Geometry check sheet. Reference: the model listing, model coordinates, mm. Round coordinates to 2 decimals unless told otherwise and drop trailing zeros. Loops run counter-clockwise (first coordinate to the right, second up) from the corner with the lowest first, then second, coordinate; pieces in that order, holes last. Notation, with made-up numbers: (-26.75, -9) - (24.25, -9) arc R9 ccw to (24.25, 3) - close; hole circle Ø7 at (-12, -6). An arc over 180 degrees is marked (long way). Answer as CSV lines item,"result". Start each with the question number.
1) Cross-section at A-A on y = 717.5. Record the boundary of the cut face in (x, z), and give its area (3 significant figures).
2) Depth check by flat-ended pin: P1, Ø5, axis at x = 27, z = 10.5, coming from the -Y side; P2, Ø5, axis at y = 1666.5, z = 7, coming from the -X side; P3, Ø12, axis at x = 13.5, y = 1499, coming from the -Z side; P4, Ø12, axis at y = 457, z = 11.5, coming from the -X side. Enter the tip coordinate at first touch or a pass-through.
3) Thickness scan on line 1 along X through (y, z) = (1412.5, 23.5); line 2 along X through (y, z) = (531.5, 17); line 3 along Z through (x, y) = (12, 785). Record the ranges inside material, lowest first.
4) Cross-section at B-B on z = 16.5. Record the boundary of the cut face in (x, y), and give its area (3 significant figures).
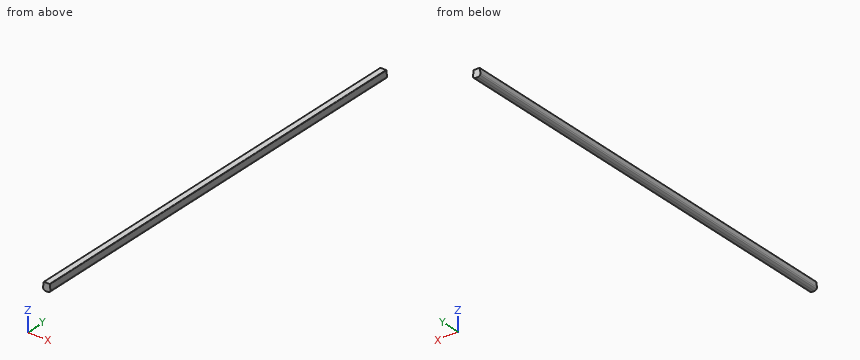
from build123d import *

# Parameters (mm, degrees)
BOSS_EXTRUDE1_DEPTH = 2133.6


with BuildPart() as part:
    # Sketch1 → Boss-Extrude1 (new body)
    with BuildSketch(Plane(origin=(0, 0, 0), x_dir=(1, 0, 0), z_dir=(0, 1, 0))):
        with BuildLine():
            Line((13.630161568, 10), (23.630161568, 10))
            ThreePointArc((23.630161568, 10), (29.962715696, 8.909575546), (34.999417241, 4.919349386))
            ThreePointArc((34.999417241, 4.919349386), (36.697471107, 1.472711464), (36.970576624, -2.359795976))
            Line((36.970576624, -2.359795976), (33.961097926, -26.870033055))
            ThreePointArc((33.961097926, -26.870033055), (33.301245719, -28.12420581), (31.976005623, -28.626294369))
            Line((31.976005623, -28.626294369), (5.284317513, -28.626294369))
            ThreePointArc((5.284317513, -28.626294369), (3.959077417, -28.12420581), (3.29922521, -26.870033055))
            Line((3.29922521, -26.870033055), (0.298191514, -2.428574989))
            ThreePointArc((0.298191514, -2.428574989), (0.53721959, 1.274672171), (2.110183266, 4.635767116))
            ThreePointArc((2.110183266, 4.635767116), (7.170061398, 8.821409583), (13.630161568, 10))
        make_face()
    extrude(amount=BOSS_EXTRUDE1_DEPTH)


solid = part.part
Answer block:
1,outline,"(0.3, 2.43) arc R10 ccw to (2.11, -4.64) arc R13 ccw to (13.63, -10) - (23.63, -10) arc R13 ccw to (35, -4.92) arc R10 ccw to (36.97, 2.36) - (33.96, 26.87) arc R2 ccw to (31.98, 28.63) - (5.28, 28.63) arc R2 ccw to (3.3, 26.87) - close"
1,area,"1,270 mm^2"
2,P1,"stops at y = 0"
2,P2,"stops at x = 0.55"
2,P3,"stops at z = -10.04"
2,P4,"stops at x = 0.68"
3,line 1,"x = 2.89 to 34.37"
3,line 2,"x = 2.09 to 35.17"
3,line 3,"z = -10.02 to 28.63"
4,outline,"(2.03, 0) - (35.23, 0) - (35.23, 2133.6) - (2.03, 2133.6) - close"
4,area,"70,900 mm^2"
